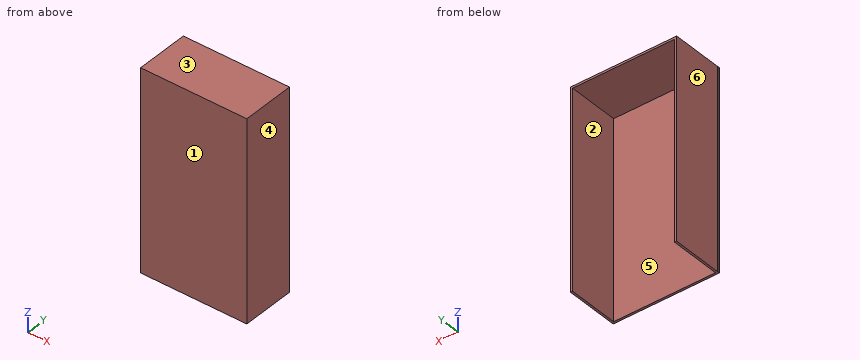
Autodesk Inventor part; units mm, degrees
ref_plane "YZ Plane" through (0, 0, 0) normal (1, 0, 0) x (0, 1, 0)
ref_plane "XZ Plane" through (0, 0, 0) normal (0, 1, 0) x (-1, 0, 0)
ref_plane "XY Plane" through (0, 0, 0) normal (0, 0, 1) x (1, 0, 0)
sketch "Sketch1" plane through (0, 0, 0) normal (0, 1, 0) x (-1, 0, 0)
  line L0 (0, 0) -> (110, 0)
  line L1 (110, 0) -> (110, -200)
  line L2 (110, -200) -> (0, -200)
  line L3 (0, -200) -> (0, 0)
  line L4 (110, -200) -> (105, -200)
  line L5 (0, -200) -> (5, -200)
  line L6 (5, -200) -> (5, -10)
  line L7 (5, -10) -> (107.5, -10)
  line L8 (105, -200) -> (105, -10)
  line L9 (5, -200) -> (7, -200)
  line L10 (7, -200) -> (7, -12)
  line L11 (7, -12) -> (103, -12)
  line L12 (7, -200) -> (7, -198)
  line L13 (7, -198) -> (103, -198)
  line L14 (103, -198) -> (103, -12)
  line L15 (103, -198) -> (105, -198)
  dimension "d0" = 110
  dimension "d1" = 200
  dimension "d2" = 5
  dimension "d3" = 5
  dimension "d4" = 190
  dimension "d5" = 2
  dimension "d6" = 188
  dimension "d7" = 96
  dimension "d8" = 2
extrude "Extrusion1" add sketch "Sketch1" along normal blind 50 contours L6 L7 L8 L15 L14 L11 L10 L2
sketch "Sketch2" plane through (0, 0, 0) normal (0, -1, 0) x (1, 0, 0)
  line L0 (-5, -10) -> (-5, -200)
  line L1 (-5, -10) -> (-105.1065, -10)
  line L2 (-105.1065, -10) -> (-105.1065, -198)
  line L3 (-105.1065, -198) -> (-5, -198)
  line L4 (-5, -198) -> (-5, -10)
  point P0 (0, 0)
extrude "Extrusion2" add sketch "Sketch2" against normal blind 2
sketch "Sketch3" plane through (-7, 0, -200) normal (-1, 0, 0) x (0, 0, 1)
  line L0 (190, 50) -> (0, 50)
  line L1 (0, 0) -> (2, 0)
  line L2 (2, 0) -> (2, 50)
  line L3 (2, 50) -> (0, 50)
  line L4 (0, 50) -> (0, 0)
  point P0 (200, 0)
  dimension "d13" = 2
extrude "Extrusion3" cut sketch "Sketch3" against normal blind 23.25
properties part number "aaaa"
Check sheet for the modelled part. Datum: model origin and axes. Units: mm. Face numbers are marked on the shaded views. A direction names the side the tool comes from. Coordinates: 2 decimals unless noted, no trailing zeros. Write each loop counter-clockwise with the first axis right and the second up, starting at its lowest first coordinate (ties: lowest second). Pieces come first, ordered by that corner, then holes. Notation, with made-up numbers: M 24.25,39.25 L 44.25,39.25 A23 ccw 44.25,65.25 Z; hole C 87.25,15.25 d4. An arc over 180 degrees is marked long. Write item = value, one per line. Start each with the question number.
1. Go/stop test with flat-tipped pins: pin 1 (1 mm diameter, centred on y = 7.5, z = -121.5, fed in from -X); pin 2 (1 mm diameter, centred on x = -66, y = 21, fed in from -Z); pin 3 (10 mm diameter, centred on x = -53.5, z = -131.5, fed in from +Y). Record where each tip stops, or that it passes through.
2. Sectioned sample at A-A (z = -102). Record the cut outline in (x, y), then the cut area to 3 significant figures.
3. Sectioned sample at C-C (x = -44.5). Record the cut outline in (y, z).
4. Sectioned sample at B-B (y = 23.5). Record the cut outline in (x, z).
5. Mould release check, pull along X, two halves, no side actions. Record for the marked faces 3, 4, 5 and 6: pulls with the +X half, pulls with the -X half, needs draft (parallel to the pull), parting line crosses it, or undercut.
6. Thickness scan on probe 1 along X at (y, z) = (22, -159); probe 2 along Y at (x, z) = (-9, -31); probe 3 along Z at (x, y) = (-82, 3). Record the ranges inside material, lowest first.
7. Tool access check on the marked faces 1 and 2. Record the directions out of +Z, -Z, +X, -X, +Y, -Y that give a thin tool (end or side, any length) a straight path to the whole face; none if there is none.
The answers:
q1.pin_1 = -105
q1.pin_2 = -12
q1.pin_3 = 2
q2.outline = M -105.11,0 L -5,0 L -5,50 L -7,50 L -7,2 L -103,2 L -103,50 L -105,50 L -105,2 L -105.11,2 Z
q2.area = 392 mm²
q3.outline = M 0,-198 L 2,-198 L 2,-12 L 50,-12 L 50,-10 L 0,-10 Z
q4.outline = M -105,-198 L -103,-198 L -103,-12 L -7,-12 L -7,-198 L -5,-198 L -5,-10 L -105,-10 Z
q5.face_3 = needs draft
q5.face_4 = pulls with the +X half
q5.face_5 = undercut
q5.face_6 = pulls with the -X half
q6.probe_1 = -105 to -103, -7 to -5
q6.probe_2 = 0 to 2
q6.probe_3 = -12 to -10
q7.face_1 = +Z, -Z, +X, -X, -Y
q7.face_2 = -Z, +Y
